Geometry check sheet. Reference: the model listing, model coordinates, mm. Give positions to 0.01 mm unless a question says otherwise; leave off trailing zeros. Order: outer loops, then holes, each group sorted by start corner. A loop starts at its lowest first (then second) coordinate and runs counter-clockwise, first axis right, second up. Notation, with made-up numbers: M 21.5,-11 L 40.5,-11 A37 cw 40.5,27 Z; hole C 31,15.5 d1. An arc over 180 degrees is marked long. Put each result on its own line as item: value. Start each with the question number.
Q1. Section check B-B on y = 268.5. Record the cut outline in (x, z).
Q2. Material ranges on L1, parallel to X at y = 400.05, z = 1.05; L2, parallel to X at y = 342.9, z = 2.75; L3, parallel to X at y = 239, z = 2.6, recorded low to high.
Q3. Go/stop test with flat-tipped pins: pin 1 (1.6 mm diameter, centred on y = 243.5, z = 2, fed in from -X); pin 2 (1.6 mm diameter, centred on x = 186, z = 2.5, fed in from +Y); pin 3 (1.6 mm diameter, centred on y = 398, z = 3, fed in from +X). Record where each tip stops, or that it passes through.
Q4. Section check D-D on z = 1.5. State how many separate pieces and enclosed holes the cut face has, then the cut area to 3 significant figures.
Q5. Section check A-A on y = 190. Record the cut outline in (x, z), then the cut area to 3 significant figures.
Q6. Section check C-C on x = -142. Record the cut outline in (y, z), then the cut area to 3 significant figures.
```python
from build123d import *

# Parameters (mm, degrees)
SKETCH1_R           = 2.5
SKETCH1_R_2         = 3.5
SKETCH1_R_3         = 2.75
BOSS_EXTRUDE1_DEPTH = 5.207


with BuildPart() as part:
    # Sketch1 → Boss-Extrude1 (new body)
    with BuildSketch(Plane.XY):
        Polygon((-189.357, 25.4), (-189.357, 0), (-157.607, 0), (-157.607, 330.2), (157.607, 330.2), (157.607, 0), (189.357, 0), (189.357, 25.4), (184.15, 25.4), (184.15, 50.8), (189.357, 50.8), (189.357, 76.2), (184.15, 76.2), (184.15, 101.6), (189.357, 101.6), (189.357, 127), (184.15, 127), (184.15, 152.4), (189.357, 152.4), (189.357, 177.8), (184.15, 177.8), (184.15, 203.2), (189.357, 203.2), (189.357, 228.6), (184.15, 228.6), (184.15, 254), (189.357, 254), (189.357, 279.4), (184.15, 279.4), (184.15, 304.8), (189.357, 304.8), (189.357, 330.2), (184.15, 330.2), (184.15, 355.6), (189.357, 355.6), (189.357, 381), (184.15, 381), (184.15, 406.4), (-184.15, 406.4), (-184.15, 381), (-189.357, 381), (-189.357, 355.6), (-184.15, 355.6), (-184.15, 330.2), (-189.357, 330.2), (-189.357, 304.8), (-184.15, 304.8), (-184.15, 279.4), (-189.357, 279.4), (-189.357, 254), (-184.15, 254), (-184.15, 228.6), (-189.357, 228.6), (-189.357, 203.2), (-184.15, 203.2), (-184.15, 177.8), (-189.357, 177.8), (-189.357, 152.4), (-184.15, 152.4), (-184.15, 127), (-189.357, 127), (-189.357, 101.6), (-184.15, 101.6), (-184.15, 76.2), (-189.357, 76.2), (-189.357, 50.8), (-184.15, 50.8), (-184.15, 25.4), align=None)
        with Locations((-170.307, 19.05)):
            Circle(SKETCH1_R, mode=Mode.SUBTRACT)
        with Locations((170.307, 19.05)):
            Circle(SKETCH1_R_2, mode=Mode.SUBTRACT)
        with Locations((-170.307, 342.9)):
            Circle(SKETCH1_R, mode=Mode.SUBTRACT)
        with Locations((-171.45, 368.05)):
            Circle(SKETCH1_R_3, mode=Mode.SUBTRACT)
        with Locations((-171.45, 400.05)):
            Circle(SKETCH1_R_3, mode=Mode.SUBTRACT)
        with Locations((170.307, 342.9)):
            Circle(SKETCH1_R, mode=Mode.SUBTRACT)
        with Locations((171.45, 368.05)):
            Circle(SKETCH1_R_3, mode=Mode.SUBTRACT)
        with Locations((171.45, 400.05)):
            Circle(SKETCH1_R_3, mode=Mode.SUBTRACT)
    extrude(amount=BOSS_EXTRUDE1_DEPTH)


solid = part.part
```
Results found:
1. outline: M -189.36,0 L -157.61,0 L -157.61,5.21 L -189.36,5.21 Z; M 157.61,0 L 189.36,0 L 189.36,5.21 L 157.61,5.21 Z
2. L1: x = -184.15 to -174.2, -168.7 to 168.7, 174.2 to 184.15
2. L2: x = -184.15 to -172.81, -167.81 to 167.81, 172.81 to 184.15
2. L3: x = -184.15 to -157.61, 157.61 to 184.15
3. pin 1: stops at x = -184.15
3. pin 2: stops at y = 381
3. pin 3: stops at x = 184.15
4. separate pieces: 1
4. enclosed holes: 8
4. area: 47,500 mm^2
5. outline: M -184.15,0 L -157.61,0 L -157.61,5.21 L -184.15,5.21 Z; M 157.61,0 L 184.15,0 L 184.15,5.21 L 157.61,5.21 Z
5. area: 276 mm^2
6. outline: M 330.2,0 L 406.4,0 L 406.4,5.21 L 330.2,5.21 Z
6. area: 397 mm^2
